The drawing under review shows one solid part. Ordinate dimensions are in mm from its lowest x, y, z. A direction names the side the tool comes from. Round coordinates to 2 decimals unless told otherwise and drop trailing zeros. Write each loop counter-clockwise with the first axis right and the second up, starting at its lowest first coordinate (ties: lowest second). Pieces come first, ordered by that corner, then holes.
Item 1: To check wall thickness, follow L1, parallel to Z at x = 10, y = 3.5; L2, parallel to X at y = 10.25, z = 12 (1 decimal); L3, parallel to X at y = 10, z = 30. State the ranges of each line that lie inside material, in increasing order.
Item 2: Add section C-C (z = 18). Give the boundary of the cut face in (x, y).
Item 3: Clearance check with flat-ended pins moving along their axes: pin 1 Ø8 at (x, z) = (8.5, 30.5) entering from -Y; pin 2 Ø1 at (x, z) = (15, 7) entering from -Y; pin 3 Ø10 at (x, z) = (12.5, 31.5) entering from +Y; pin 4 Ø8 at (y, z) = (13, 6.5) entering from +X. State where each tip first meets the part, or that it passes through.
Item 4: Add section D-D (z = 33.5). Give the boundary of the cut face in (x, y).
Item 5: Machinability: for the marked faces 1 and 2, which of the approach directions +Z, -Z, +X, -X, +Y, -Y give a long, thin tool a straight path to every point of the face, cutting with its end or side? Answer none if there is none.
Item 6: Add section A-A (y = 10). Give the boundary of the cut face in (x, z).
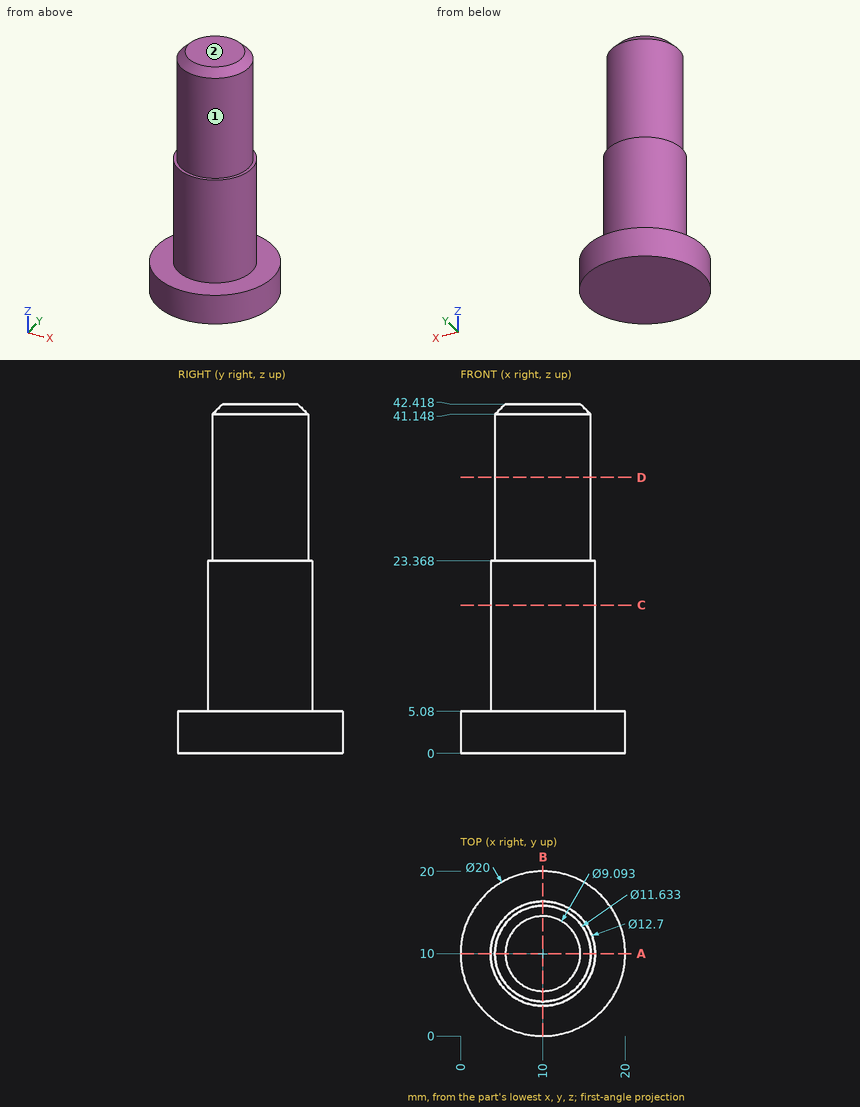
Numbers:
1. L1: z = 0 to 5.08
1. L2: x = 3.7 to 16.3
1. L3: x = 4.18 to 15.82
2. outline: circle Ø12.7 at (10, 10)
3. pin 1: stops at y = 4.18
3. pin 2: stops at y = 5.52
3. pin 3: stops at y = 15.82
3. pin 4: stops at x = 20
4. outline: circle Ø11.63 at (10, 10)
5. face 1: +Z
5. face 2: +Z, +X, -X, +Y, -Y
6. outline: (0, 0) - (20, 0) - (20, 5.08) - (16.35, 5.08) - (16.35, 23.37) - (15.82, 23.37) - (15.82, 41.15) - (14.55, 42.42) - (5.45, 42.42) - (4.18, 41.15) - (4.18, 23.37) - (3.65, 23.37) - (3.65, 5.08) - (0, 5.08) - close
